Could you check a few things on this model? Use its own coordinates, in mm. Face numbers are marked on the shaded views. A direction names the side the tool comes from. Give positions to 0.01 mm unless a question says otherwise; leave off trailing zeros. Order: outer loops, then holes, each group sorted by start corner. A loop starts at its lowest first (then second) coordinate and runs counter-clockwise, first axis right, second up. Notation, with made-up numbers: M 70.25,66 L 92.25,66 A27 ccw 92.25,84 Z; hole C 26,40.5 d3. An arc over 180 degrees is marked long. Answer in a Markdown table with one row per item. Add a question column.
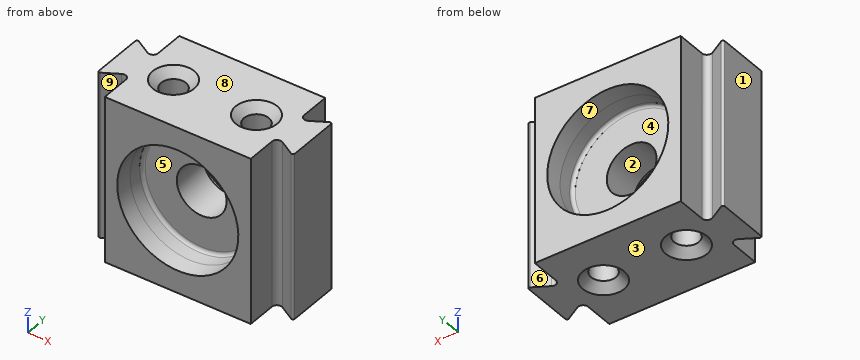
```python
from build123d import *

# Parameters (mm, degrees)
BOSS_EXTRUDE1_DEPTH = 20
SKETCH2_R           = 7.2
CUT_EXTRUDE1_DEPTH  = 4
SKETCH3_R           = 3
CUT_EXTRUDE2_DEPTH  = 26.061299571
SKETCH4_R           = 1.5
CUT_EXTRUDE3_DEPTH  = 36.603512784
CHAMFER1_SIZE       = 1
FILLET1_R           = 0.4
CHAMFER2_SIZE       = 0.1
CHAMFER2_SIZE2      = 2
CHAMFER3_SIZE       = 2
CHAMFER3_SIZE2      = 0.1


with BuildPart() as part:
    # Sketch1 → Boss-Extrude1 (new body)
    with BuildSketch(Plane.XY):
        with BuildLine():
            Line((-8.092893219, -26.668003347), (0.707106781, -26.668003347))
            Line((0.707106781, -26.668003347), (0.707106781, -14.203901732))
            Line((0.707106781, -14.203901732), (-8.092893219, -14.203901732))
            Line((-8.092893219, -14.203901732), (-8.092893219, -17.743132217))
            ThreePointArc((-8.092893219, -17.743132217), (-8.392893219, -18.262747459), (-8.992893219, -18.262747459))
            Line((-8.992893219, -18.262747459), (-10.792893219, -17.223516975))
            ThreePointArc((-10.792893219, -17.223516975), (-10.992893219, -17.223516975), (-11.092893219, -17.396722055))
            Line((-11.092893219, -17.396722055), (-11.092893219, -23.475183024))
            ThreePointArc((-11.092893219, -23.475183024), (-10.992893219, -23.648388105), (-10.792893219, -23.648388105))
            Line((-10.792893219, -23.648388105), (-8.992893219, -22.609157621))
            ThreePointArc((-8.992893219, -22.609157621), (-8.392893219, -22.609157621), (-8.092893219, -23.128772863))
            Line((-8.092893219, -23.128772863), (-8.092893219, -26.668003347))
        make_face()
    extrude(amount=-BOSS_EXTRUDE1_DEPTH)

    # Mirror1: part across plane


with BuildPart() as part_1:
    add(part.part)
    add(part.part.mirror(Plane(origin=(0.707106781, -26.668003347, -20), x_dir=(0, 0, 1), z_dir=(1, 0, 0))))

    # Sketch2 → Cut-Extrude1 (cut)
    with BuildSketch(Plane(origin=(0, -14.203901732, 0), x_dir=(1, 0, 0), z_dir=(0, 1, 0))):
        with Locations(Location((0.707106781, 10, 0), (0, 0, 270))):
            Circle(SKETCH2_R)
    cut_extrude1 = extrude(amount=-CUT_EXTRUDE1_DEPTH, mode=Mode.SUBTRACT)

    # Mirror2: Cut-Extrude1 across plane
    add(cut_extrude1.mirror(Plane(origin=(0, -20.43595254, 0), x_dir=(0, 0, 1), z_dir=(0, -1, 0))), mode=Mode.SUBTRACT)

    # Sketch3 → Cut-Extrude2 (cut, through all)
    with BuildSketch(Plane(origin=(0, -18.203901732, 0), x_dir=(1, 0, 0), z_dir=(0, 1, 0))):
        with Locations(Location((0.707106781, 10, 0), (0, 0, 270))):
            Circle(SKETCH3_R)
    extrude(amount=-CUT_EXTRUDE2_DEPTH, mode=Mode.SUBTRACT)

    # Sketch4 → Cut-Extrude3 (cut, through all)
    with BuildSketch(Plane(origin=(0, 0, -20), x_dir=(-1, 0, 0), z_dir=(0, 0, -1))):
        with Locations((4.292893219, -20.43595254)):
            Circle(SKETCH4_R)
        with Locations(Location((-5.707106781, -20.43595254, 0), (0, 0, 180))):
            Circle(SKETCH4_R)
    extrude(amount=-CUT_EXTRUDE3_DEPTH, mode=Mode.SUBTRACT)

    # Chamfer1
    chamfer1_edges = [part_1.edges().sort_by_distance(p)[0] for p in [
        (-2.792893219, -20.43595254, 0),
        (-2.792893219, -20.43595254, -20),
        (4.207106781, -20.43595254, 0),
        (4.207106781, -20.43595254, -20),
    ]]
    chamfer(chamfer1_edges, length=CHAMFER1_SIZE)

    # Fillet1
    fillet1_edges = [part_1.edges().sort_by_distance(p)[0] for p in [
        (0.707106781, -18.203901732, -17.2),
        (0.707106781, -22.668003347, -17.2),
    ]]
    fillet(fillet1_edges, radius=FILLET1_R)

    # Chamfer2
    chamfer2_edges = [part_1.edges().sort_by_distance(p)[0] for p in [
        (0.707106781, -14.203901732, -17.2),
    ]]
    chamfer2_side = [part_1.faces().sort_by_distance(p)[0] for p in [
        (-7.826480006, -14.203901732, -10),
    ]]
    chamfer(chamfer2_edges, length=CHAMFER2_SIZE, length2=CHAMFER2_SIZE2, reference=chamfer2_side[0])

    # Chamfer3
    chamfer3_edges = [part_1.edges().sort_by_distance(p)[0] for p in [
        (0.707106781, -26.668003347, -17.2),
    ]]
    chamfer3_side = [part_1.faces().sort_by_distance(p)[0] for p in [
        (0.707106781, -24.868003347, -17.2),
    ]]
    chamfer(chamfer3_edges, length=CHAMFER3_SIZE, length2=CHAMFER3_SIZE2, reference=chamfer3_side[0])


solid = part_1.part
```
1. If I drill on line 1 along X through (y, z) = (-17.35, -10); line 2 along X through (y, z) = (-23.75, -10); line 3 along Y through (x, z) = (-4.25, -1.5), over which ranges is the centre line in solid material (lowest first)? Write a range as [from, to].
2. Will these pins go through, and if not, where does the flat tip stop? P1, Ø1.5, axis at x = 6, z = -8.5, coming from the -Y side; P2, Ø4, axis at x = -4.29, y = -20.44, coming from the +Z side (3 decimals); P3, Ø3, axis at x = 3.5, z = -6.5, coming from the +Y side.
3. Suppose I cut it at A-A on z = -2. List the corners of the cut face in (x, y) for me, plus the area to 3 significant figures.
4. For the marked faces 5, 6, 7, 8 and 9, which set-ups out of +Z, -Z, +X, -X, +Y, -Y let a thin tool reach every point of the face, with its end or its side?
5. Suppose I cut it at B-B on y = -16.75. List the corners of the cut face in (x, z) for me.
6. Suppose I cut it at C-C on y = -21. Count the separate pieces of the cut face and the enclosed holes in it, plus the area to 3 significant figures.
7. Thinking about a two-plate mould opening in Z: for the marked faces 1, 2, 3 and 4, which applies, pulls with the +Z half, pulls with the -Z half, needs draft (parallel to the pull), parting line crosses it, or undercut?
Findings below:
| question | item | result |
|---|---|---|
| 1 | line 1 | [-11.09, -10.57], [-8.09, -6.49], [7.91, 9.51], [11.99, 12.5] |
| 1 | line 2 | [-8.09, -6.49], [7.91, 9.51] |
| 1 | line 3 | [-26.67, -21.94], [-18.94, -14.2] |
| 2 | P1 | y = -22.67 |
| 2 | P2 | z = -0.495 |
| 2 | P3 | y = -18.2 |
| 3 | outline | M -11.09,-23.48 A0.2 ccw -10.79,-23.65 L -8.99,-22.61 A0.6 cw -8.09,-23.13 L -8.09,-26.67 L 9.51,-26.67 L 9.51,-23.13 A0.6 cw 10.41,-22.61 L 12.21,-23.65 A0.2 ccw 12.51,-23.48 L 12.51,-17.4 A0.2 ccw 12.21,-17.22 L 10.41,-18.26 A0.6 cw 9.51,-17.74 L 9.51,-14.2 L -8.09,-14.2 L -8.09,-17.74 A0.6 cw -8.99,-18.26 L -10.79,-17.22 A0.2 ccw -11.09,-17.4 Z; hole C -4.29,-20.44 d3; hole C 5.71,-20.44 d3 |
| 3 | area | 236 mm2 |
| 4 | face 5 | -Y |
| 4 | face 6 | +Z, -Z, +Y |
| 4 | face 7 | +Y |
| 4 | face 8 | +Z, +X, -X, +Y, -Y |
| 4 | face 9 | +Z, -Z, -Y |
| 5 | outline | M -8.09,-20 L 9.51,-20 L 9.51,0 L -8.09,0 Z; hole C 0.71,-10 d14.4 |
| 6 | separate pieces | 3 |
| 6 | enclosed holes | 1 |
| 6 | area | 328 mm2 |
| 7 | face 1 | needs draft |
| 7 | face 2 | undercut |
| 7 | face 3 | pulls with the -Z half |
| 7 | face 4 | undercut |
